Input: part model. Units: mm. Frame: model coordinates. Face numbers are marked on the shaded views. A direction names the side the tool comes from. Coordinates: 2 decimals unless noted, no trailing zeros. Loops run counter-clockwise (first coordinate to the right, second up) from the corner with the lowest first, then second, coordinate; pieces in that order, holes last. Notation, with made-up numbers: M 76,83 L 101,83 A25 cw 101,100 Z; hole C 64,48 d7. An arc over 180 degrees is marked long. Use a Markdown table: item, result. Add a question column.
1. Pin query (flat end, axial travel): pin 1 (10 mm diameter, centred on x = -31.5, z = -1, fed in from -Y); pin 2 (5.5 mm diameter, centred on x = -3.5, y = 2, fed in from +Z); pin 3 (4 mm diameter, centred on x = -45, z = 10.5, fed in from +Y); pin 4 (9 mm diameter, centred on y = 12.5, z = -21.5, fed in from +X). Return the tip coordinate at first contact, or that it passes through.
2. Section C-C on y = 17.5. Output: boundary loops of the cut face in (x, z), then the cut area to 3 significant figures.
3. Line query: L1, parallel to X at y = 2, z = -11.5; L2, parallel to Z at x = 45, y = 1; L3, parallel to Y at x = 2.5, z = 1. Output: solid intervals per line, ascending. Write a range as [from, to].
4. Section A-A on z = -21. Output: boundary loops of the cut face in (x, y).
5. Draft query along X for the marked faces 4, 5, 6 and 7. Return one class per face: +X half, -X half, draft (parallel to the pull), parting line (faces both ways), or undercut.
6. Set-up query: the marked faces 1, 2 and 3. Return all of +Z, -Z, +X, -X, +Y, -Y with unobstructed straight access to the full face (end or side cutting, diameter ignored); none if empty.
7. Section D-D on z = 11. Output: boundary loops of the cut face in (x, y).
8. Section B-B on x = -45. Output: boundary loops of the cut face in (y, z), then the cut area to 3 significant figures.
```python
from build123d import *

# Parameters (mm, degrees)
EXTRUDE_1_DEPTH     = 5
FILLET_1_R          = 10
EXTRUDE_2_DEPTH     = 8
FILLET_4_R          = 3
SKETCH_3_R          = 1.5
CUT_EXTRUDE_1_DEPTH = 5
CHAMFER_1_SIZE      = 10
FILLET_5_R          = 3
CUT_EXTRUDE_2_DEPTH = 5
FILLET_6_R          = 2
FILLET_7_R          = 2
CHAMFER_2_SIZE      = 15
FILLET_8_R          = 3
SKETCH_6_R          = 2.15
CUT_EXTRUDE_3_DEPTH = 52
CHAMFER_3_SIZE      = 3


with BuildPart() as part:
    # 草图1 → 凸台-拉伸1 (new body)
    with BuildSketch(Plane(origin=(0, 0, 0), x_dir=(1, 0, 0), z_dir=(0, 1, 0))):
        Polygon((-50, -25), (-33.660254038, -25), (-25, -10), (25, -10), (33.660254038, -25), (50, -25), (50, 25), (-50, 25), align=None)
    extrude(amount=EXTRUDE_1_DEPTH)

    # 圆角1
    fillet_1_edges = [part.edges().sort_by_distance(p)[0] for p in [
        (-25, 2.5, 10),
        (-33.660254038, 2.5, 25),
        (33.660254038, 2.5, 25),
        (25, 2.5, 10),
    ]]
    fillet(fillet_1_edges, radius=FILLET_1_R)

    # 草图2 → 凸台-拉伸2 (add)
    with BuildSketch(Plane(origin=(0, 0, -25), x_dir=(-1, 0, 0), z_dir=(0, 0, -1))):
        Polygon((-15, 33), (-15, 5), (-11, 5), (-11, 27.2), (0, 27.2), (11, 27.2), (11, 5), (15, 5), (15, 33), align=None)
    extrude(amount=-EXTRUDE_2_DEPTH)

    # 圆角4
    fillet_4_edges = [part.edges().sort_by_distance(p)[0] for p in [
        (15, 33, -21),
        (-15, 33, -21),
    ]]
    fillet(fillet_4_edges, radius=FILLET_4_R)

    # 草图3 → 切除-拉伸1 (cut)
    with BuildSketch(Plane.XZ):
        with Locations(Location((-45, 10.5, 0), (0, 0, 270))):
            Circle(SKETCH_3_R)
        with Locations(Location((-45, -9.5, 0), (0, 0, 270))):
            Circle(SKETCH_3_R)
        with Locations(Location((45, -9.5, 0), (0, 0, 90))):
            Circle(SKETCH_3_R)
        with Locations(Location((45, 10.5, 0), (0, 0, 90))):
            Circle(SKETCH_3_R)
    extrude(amount=-CUT_EXTRUDE_1_DEPTH, mode=Mode.SUBTRACT)

    # 倒角1
    chamfer_1_edges = [part.edges().sort_by_distance(p)[0] for p in [
        (-50, 2.5, -25),
        (50, 2.5, -25),
    ]]
    chamfer(chamfer_1_edges, length=CHAMFER_1_SIZE)

    # 圆角5
    fillet_5_edges = [part.edges().sort_by_distance(p)[0] for p in [
        (-50, 2.5, 25),
        (50, 2.5, 25),
    ]]
    fillet(fillet_5_edges, radius=FILLET_5_R)

    # 草图4 → 切除-拉伸2 (cut)
    with BuildSketch(Plane(origin=(0, 5, 0), x_dir=(1, 0, 0), z_dir=(0, 1, 0))):
        Polygon((-35, 16), (-35, -10), (-24.607695155, -4), (-24.607695155, 10), align=None)
        Polygon((24.607695155, -4), (24.607695155, 10), (35, 16), (35, -10), align=None)
    extrude(amount=-CUT_EXTRUDE_2_DEPTH, mode=Mode.SUBTRACT)

    # 圆角6
    fillet_6_edges = [part.edges().sort_by_distance(p)[0] for p in [
        (-35, 2.5, -16),
        (-24.607695155, 2.5, -10),
        (-24.607695155, 2.5, 4),
        (-35, 2.5, 10),
    ]]
    fillet(fillet_6_edges, radius=FILLET_6_R)

    # 圆角7
    fillet_7_edges = [part.edges().sort_by_distance(p)[0] for p in [
        (35, 2.5, 10),
        (24.607695155, 2.5, 4),
        (24.607695155, 2.5, -10),
        (35, 2.5, -16),
    ]]
    fillet(fillet_7_edges, radius=FILLET_7_R)

    # 倒角2
    chamfer_2_edges = [part.edges().sort_by_distance(p)[0] for p in [
        (15, 5, -21),
        (-15, 5, -21),
    ]]
    chamfer(chamfer_2_edges, length=CHAMFER_2_SIZE)

    # 圆角8
    fillet_8_edges = [part.edges().sort_by_distance(p)[0] for p in [
        (-11, 5, -21),
        (-11, 27.2, -21),
        (11, 27.2, -21),
        (11, 5, -21),
    ]]
    fillet(fillet_8_edges, radius=FILLET_8_R)

    # 草图6 → 切除-拉伸3 (cut)
    with BuildSketch(Plane(origin=(0, 33, 0), x_dir=(1, 0, 0), z_dir=(0, 1, 0))):
        with Locations(Location((0, 21, 0), (0, 0, 270))):
            Circle(SKETCH_6_R)
    extrude(amount=-CUT_EXTRUDE_3_DEPTH, mode=Mode.SUBTRACT)

    # 倒角3
    chamfer_3_edges = [part.edges().sort_by_distance(p)[0] for p in [
        (19, 5, -17),
        (-19, 5, -17),
    ]]
    chamfer(chamfer_3_edges, length=CHAMFER_3_SIZE)


solid = part.part
```
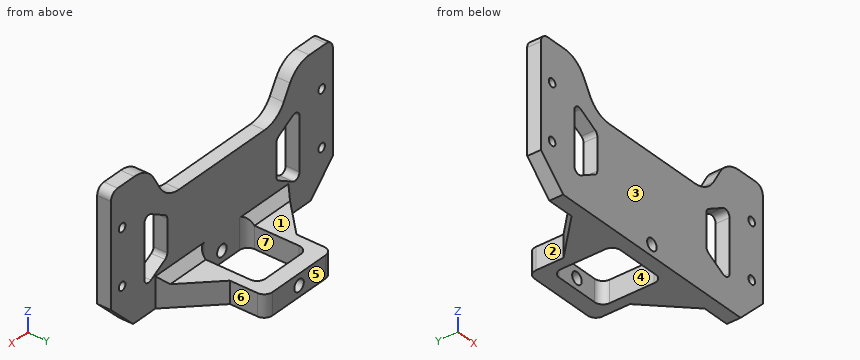
Answers below:
| question | item | result |
|---|---|---|
| 1 | pin 1 | stops at y = 0 |
| 1 | pin 2 | stops at z = 10 |
| 1 | pin 3 | stops at y = 5 |
| 1 | pin 4 | stops at x = 27 |
| 2 | outline | M -17.5,-25 L -11,-25 L -11,-17 L -17.5,-17 Z; M 11,-25 L 17.5,-25 L 17.5,-17 L 11,-17 Z |
| 2 | area | 104 mm² |
| 3 | L1 | x = [-50, -35], [-27.21, 27.21], [35, 50] |
| 3 | L2 | z = [-20, -11], [-8, 9], [12, 25] |
| 3 | L3 | y = [0, 5] |
| 4 | outline | M -44,0 L -2.15,0 L -2.15,5 L -8,5 A3 cw -11,8 L -11,24.2 A3 cw -8,27.2 L -2.15,27.2 L -2.15,33 L -12,33 A3 ccw -15,30 L -15,20 L -30,5 L -44,5 Z; M 2.15,0 L 44,0 L 44,5 L 30,5 L 15,20 L 15,30 A3 ccw 12,33 L 2.15,33 L 2.15,27.2 L 8,27.2 A3 cw 11,24.2 L 11,8 A3 cw 8,5 L 2.15,5 Z |
| 5 | face 4 | undercut |
| 5 | face 5 | draft |
| 5 | face 6 | +X half |
| 5 | face 7 | undercut |
| 6 | face 1 | +Z, +X, -X, +Y |
| 6 | face 2 | +Z, -Z, -X, +Y |
| 6 | face 3 | +Z, -Z, +X, -X, -Y |
| 7 | outline | M -50,0 L -46.41,0 L -46.41,5 L -50,5 Z; M -43.59,0 L -23.59,0 L -23.59,5 L -43.59,5 Z; M 23.59,0 L 43.59,0 L 43.59,5 L 23.59,5 Z; M 46.41,0 L 50,0 L 50,5 L 46.41,5 Z |
| 8 | outline | M 0,-20 L 5,-20 L 5,-11 L 0,-11 Z; M 0,-8 L 5,-8 L 5,9 L 0,9 Z; M 0,12 L 5,12 L 5,25 L 0,25 Z |
| 8 | area | 195 mm² |
